Work out the finished part from the listing and answer in its coordinate system (mm). A direction names the side the tool comes from. Give positions to 0.01 mm unless a question says otherwise; leave off trailing zeros. Loops run counter-clockwise (first coordinate to the right, second up) from the corner with the lowest first, then second, coordinate; pieces in that order, holes last. Notation, with made-up numbers: (54.5, 30.25) - (80.5, 30.25) arc R22 cw to (80.5, 37.25) - close; hole circle Ø10 at (38, 66). An arc over 180 degrees is marked (long way). Use CSV: the item, a comma, the result in double quotes.
from build123d import *

# Parameters (mm, degrees)
SKETCH_2_W          = 50
SKETCH_2_H          = 50
EXTRUDE_1_DEPTH     = 13
SKETCH_3_W          = 8
SKETCH_3_H          = 50
CUT_EXTRUDE_1_DEPTH = 10
SKETCH_4_W          = 50
SKETCH_4_H          = 4
CUT_EXTRUDE_2_DEPTH = 4
CUT_EXTRUDE_4_DEPTH = 4
CUT_EXTRUDE_5_DEPTH = 4
CUT_EXTRUDE_6_DEPTH = 4
CUT_EXTRUDE_7_DEPTH = 4
CUT_EXTRUDE_8_DEPTH = 38.669616404


with BuildPart() as part:
    # 草图2 → 凸台-拉伸1 (new body)
    with BuildSketch(Plane(origin=(0, 0, 0), x_dir=(1, 0, 0), z_dir=(0, 1, 0))):
        Rectangle(SKETCH_2_W, SKETCH_2_H)
    extrude(amount=EXTRUDE_1_DEPTH)

    # 草图3 → 切除-拉伸1 (cut)
    with BuildSketch(Plane(origin=(0, 13, 0), x_dir=(1, 0, 0), z_dir=(0, 1, 0))):
        Rectangle(SKETCH_3_W, SKETCH_3_H)
    extrude(amount=-CUT_EXTRUDE_1_DEPTH, mode=Mode.SUBTRACT)

    # 草图4 → 切除-拉伸2 (cut)
    with BuildSketch(Plane(origin=(0, 13, 0), x_dir=(1, 0, 0), z_dir=(0, 1, 0))):
        Rectangle(SKETCH_4_W, SKETCH_4_H)
    extrude(amount=-CUT_EXTRUDE_2_DEPTH, mode=Mode.SUBTRACT)

    # 草图5 → 切除-拉伸4 (cut)
    with BuildSketch(Plane(origin=(0, 13, 0), x_dir=(1, 0, 0), z_dir=(0, 1, 0))):
        Polygon((-1.282274203, 2.220964068), (1.282274203, -2.220964068), (-26.199867727, -18.087786109), (-28.764416132, -13.645857973), align=None)
    extrude(amount=-CUT_EXTRUDE_4_DEPTH, mode=Mode.SUBTRACT)

    # 草图7 → 切除-拉伸5 (cut)
    with BuildSketch(Plane(origin=(0, 13, 0), x_dir=(1, 0, 0), z_dir=(0, 1, 0))):
        Polygon((-1.881421881, -1.881421881), (1.881421881, 1.881421881), (-24.724588242, 28.487432004), (-28.487432004, 24.724588242), align=None)
    extrude(amount=-CUT_EXTRUDE_5_DEPTH, mode=Mode.SUBTRACT)

    # 草图8 → 切除-拉伸6 (cut)
    with BuildSketch(Plane(origin=(0, 13, 0), x_dir=(1, 0, 0), z_dir=(0, 1, 0))):
        Polygon((-1.54081376, -1.54081376), (1.54081376, 1.54081376), (29.908508957, -26.826881437), (26.826881437, -29.908508957), align=None)
    extrude(amount=-CUT_EXTRUDE_6_DEPTH, mode=Mode.SUBTRACT)

    # 草图9 → 切除-拉伸7 (cut)
    with BuildSketch(Plane(origin=(0, 13, 0), x_dir=(1, 0, 0), z_dir=(0, 1, 0))):
        Polygon((-1.309113008, 2.267450243), (1.309113008, -2.267450243), (34.209084597, 16.72735721), (31.590858581, 21.262257696), align=None)
    extrude(amount=-CUT_EXTRUDE_7_DEPTH, mode=Mode.SUBTRACT)

    # 草图10 → 切除-拉伸8 (cut, through all)
    with BuildSketch(Plane(origin=(0, 13, 0), x_dir=(1, 0, 0), z_dir=(0, 1, 0))):
        Polygon((-25, -11.472471306), (-17.189877667, -25), (-25, -25), align=None)
        Polygon((25, 11.410489739), (17.154092593, 25), (25, 25), align=None)
    extrude(amount=-CUT_EXTRUDE_8_DEPTH, mode=Mode.SUBTRACT)


solid = part.part
Item 1: For faces 4 (the flat face through (-15.516, 11.028, -11.753)), 5 (the flat face through (4, 8, 0)), 6 (the flat face through (11, 13, -17)), 7 (the flat face through (0, 0, 0)), 8 (the flat face through (-16, 11, -2)), determine the directions among +Z, -Z, +X, -X, +Y, -Y from which every point of the face is accessible in a straight line to the end or side of a thin tool.
Determined:
face 4,"+Y"
face 5,"+Z, -Z, +Y"
face 6,"+Z, -Z, +X, -X, +Y"
face 7,"+Z, -Z, +X, -X, -Y"
face 8,"+X, -X, +Y"
Item 2: Given P1, Ø4.5, axis at x = -19.5, y = 11, coming from the +Z side, flat-ended and moving along its own axis, determine where the tip first touches the part or whether it passes through.
Determined:
P1,"stops at z = 24.9"
Item 3: Find the intervals of material crossed by line 1 (X direction, y = 8.25, z = 7); line 2 (X direction, y = 12, z = -10); line 3 (Z direction, x = -7.5, y = 9.5), in increasing order.
Determined:
line 1,"x = -25 to -4, 4 to 25"
line 2,"x = -25 to -13.76, -6.24 to -4, 4 to 12.08, 22.56 to 25"
line 3,"z = -25 to -11.26, -3.74 to -2, 7.29 to 25"
Item 4: A cutting plane is placed at A-A on y = 10.75. Determine the outline of the cut face in (x, z), and give its area (3 significant figures).
Determined:
outline,"(-25, -21.24) - (-5.76, -2) - (-25, -2) - close; (-25, 2) - (-8.59, 2) - (-25, 11.47) - close; (-22.44, 15.91) - (-4, 5.27) - (-4, 25) - (-17.19, 25) - close; (-21.24, -25) - (-4, -25) - (-4, -7.76) - close; (4, -25) - (17.15, -25) - (22.38, -15.95) - (4, -5.33) - close; (4, 7.08) - (21.92, 25) - (4, 25) - close; (5.08, 2) - (25, 2) - (25, 21.92) - close; (8.7, -2) - (25, -11.41) - (25, -2) - close"
area,"1,330 mm²"
Item 5: A cutting plane is placed at C-C on y = 6.5. Determine the outline of the cut face in (x, z), and give its area (3 significant figures).
Determined:
outline,"(-25, -25) - (-4, -25) - (-4, 25) - (-17.19, 25) - (-25, 11.47) - close; (4, -25) - (17.15, -25) - (25, -11.41) - (25, 25) - (4, 25) - close"
area,"1,990 mm²"
Item 6: The mould has two halves that part along Z. Classify faces 1 (the flat face through (0, 3, 0)), 2 (the flat face through (14.9, 11.03, 11.82)), 3 (the flat face through (13.085, 11.028, 16.166)): pulls with the +Z half, pulls with the -Z half, needs draft (parallel to the pull), parting line crosses it, or undercut.
Determined:
face 1,"needs draft"
face 2,"undercut"
face 3,"undercut"
Item 7: A cutting plane is placed at B-B on z = -1. Determine the outline of the cut face in (x, y), and give its area (3 significant figures).
Determined:
outline,"(-25, 0) - (25, 0) - (25, 9) - (4, 9) - (4, 3) - (-4, 3) - (-4, 9) - (-25, 9) - close"
area,"402 mm²"
Item 8: A cutting plane is placed at D-D on x = 19.5. Determine the outline of the cut face in (y, z), and give its area (3 significant figures).
Determined:
outline,"(0, -20.94) - (13, -20.94) - (13, -14.28) - (9, -14.28) - (9, -8.24) - (13, -8.24) - (13, -2) - (9, -2) - (9, 2) - (13, 2) - (13, 16.42) - (9, 16.42) - (9, 22.58) - (13, 22.58) - (13, 25) - (0, 25) - close"
area,"532 mm²"
